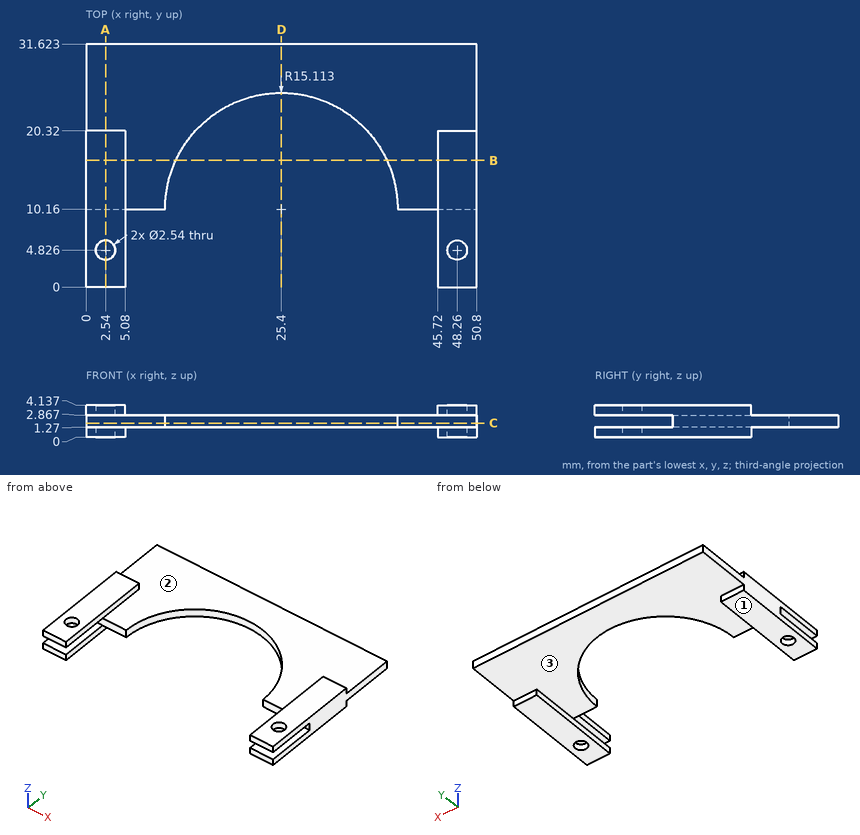
For this review, use the dimensioned drawing (mm, ordinates from the lowest corner) and the shaded views. Give positions to 0.01 mm unless a question says otherwise; leave off trailing zeros. Order: outer loops, then holes, each group sorted by start corner. A loop starts at its lowest first (then second) coordinate and runs counter-clockwise, first axis right, second up. Notation, with made-up numbers: M -32.5,12 L 20.5,12 A24 ccw 20.5,43 Z; hole C -10,37.5 d5. An arc over 180 degrees is marked long. Use one line per item in the form item = value. Start each with the question number.
Item 1: To check wall thickness, follow line 1 along X through (y, z) = (16, 3.05); line 2 along Y through (x, z) = (2.54, 3.7); line 3 along Z through (x, y) = (4.5, 4). State the ranges of each line that lie inside material, in increasing order. Write a range as from..to.
Item 2: We need section B-B on y = 16.5. Give the boundary of the cut face in (x, z), plus the area to 3 significant figures.
Item 3: We need section A-A on x = 2.54. Give the boundary of the cut face in (y, z).
Item 4: The part is to be moulded in two halves that separate along X. For the marked faces 1, 2 and 3, say which applies: pulls with the +X half, pulls with the -X half, needs draft (parallel to the pull), parting line crosses it, or undercut.
Item 5: We need section D-D on x = 25.4. Give the boundary of the cut face in (y, z), plus the area to 3 significant figures.
Item 6: We need section C-C on z = 1.8. Give the boundary of the cut face in (x, y), plus the area to 3 significant figures.
Item 7: Insertion check: pin 1 Ø1 at (x, y) = (33.5, 26) entering from -Z; pin 2 Ø0.5 at (x, z) = (44, 2) entering from -Y. Each pin has a flat end and moves straight along its axis. Give the tip position at first contact, or say it passes through.
Completed:
q1.line_1 = 0..5.08, 45.72..50.8
q1.line_2 = 0..3.56, 6.1..20.32
q1.line_3 = 0..1.27, 2.87..4.14
q2.outline = M 0,0 L 5.08,0 L 5.08,1.27 L 11.68,1.27 L 11.68,2.87 L 5.08,2.87 L 5.08,4.14 L 0,4.14 Z; M 39.12,1.27 L 45.72,1.27 L 45.72,0 L 50.8,0 L 50.8,4.14 L 45.72,4.14 L 45.72,2.87 L 39.12,2.87 Z
q2.area = 63.1 mm²
q3.outline = M 0,0 L 3.56,0 L 3.56,1.27 L 0,1.27 Z; M 0,2.87 L 3.56,2.87 L 3.56,4.14 L 0,4.14 Z; M 6.1,0 L 20.32,0 L 20.32,1.27 L 31.62,1.27 L 31.62,2.87 L 20.32,2.87 L 20.32,4.14 L 6.1,4.14 L 6.1,2.87 L 10.16,2.87 L 10.16,1.27 L 6.1,1.27 Z
q4.face_1 = needs draft
q4.face_2 = undercut
q4.face_3 = undercut
q5.outline = M 25.27,1.27 L 31.62,1.27 L 31.62,2.87 L 25.27,2.87 Z
q5.area = 10.1 mm²
q6.outline = M 0,10.16 L 10.29,10.16 A15.11 cw 40.51,10.16 L 50.8,10.16 L 50.8,31.62 L 0,31.62 Z
q6.area = 732 mm²
q7.pin_1 = 1.27
q7.pin_2 = 10.16
